```python
from build123d import *

# Parameters (mm, degrees)
F0_W          = 87.5
F0_H          = 92
F1_DEPTH      = 42
F1_TAPER      = 4
F1_DEPTH_BACK = 33
F5_SIZE       = 5
F6_T1_DEPTH   = 58.7168298797
F6_T3_DEPTH   = 62.7898982715
F6_T5_DEPTH   = 62.7898982715
F6_T7_DEPTH   = 62.7898982715
F6_T9_DEPTH   = 62.7898982715
F7_T1_DEPTH   = 103.6905771188
F7_T3_DEPTH   = 44.0479092504
F7_T5_DEPTH   = 44.0479092504
F7_T7_DEPTH   = 108.1905771188
F7_T9_DEPTH   = 44.0479092503
F7_T11_DEPTH  = 44.0479092503


# Not quite as in the source:
# - a fillet or chamfer that OpenCascade refuses, or shapes differently, is made with other operations: its cross-section is extruded or revolved along the edge and cut away or added


with BuildPart() as f1:
    # F0 (on Top) → F1 (new body, two sides)
    with BuildSketch(Plane.XY) as f1_sk:
        with Locations((0, -1.4119595289)):
            Rectangle(F0_W, F0_H)
    extrude(amount=F1_DEPTH, taper=F1_TAPER)
    extrude(f1_sk.sketch, amount=-F1_DEPTH_BACK)

    # F5
    f5_edges = [f1.edges().sort_by_distance(p)[0] for p in [
        (0, -44.475033, 42),
        (40.813074, -1.41196, 42),
        (0, 41.651114, 42),
        (-40.813074, -1.41196, 42),
    ]]
    chamfer(f5_edges, length=F5_SIZE)

    # F6: chamfer of 5 on 8 edges, made by hand

    # F6_s2 → F6_t1 (cut)
    with BuildSketch(Plane.XY.offset(-45.8584149398)):
        Polygon((43.75, 39.5880404711), (38.75, 44.5880404711), (43.75, 44.5880404711), align=None)
        Polygon((-43.75, 39.5880404711), (-38.75, 44.5880404711), (-43.75, 44.5880404711), align=None)
        Polygon((-38.75, -47.4119595289), (-43.75, -42.4119595289), (-43.75, -47.4119595289), align=None)
        Polygon((38.75, -47.4119595289), (43.75, -42.4119595289), (43.75, -47.4119595289), align=None)
    extrude(amount=F6_T1_DEPTH, mode=Mode.SUBTRACT)

    # F6_s4 → F6_t3 (cut)
    with BuildSketch(Plane(origin=(-1.3320626645, -1.3320626645, -19.0493835976), x_dir=(-0.7071067812, 0.7071067812, 0), z_dir=(0.0695873743, 0.0695873743, 0.9951458158))):
        Polygon((-6.1163179384, 60.6385318402), (0.9375251077, 60.6385318402), (-2.5893964153, 64.1483330365), align=None)
    extrude(amount=F6_T3_DEPTH, mode=Mode.SUBTRACT)

    # F6_s6 → F6_t5 (cut)
    with BuildSketch(Plane(origin=(1.3320626645, -1.3320626645, -19.0493835976), x_dir=(-0.7071067812, -0.7071067812, 0), z_dir=(-0.0695873743, 0.0695873743, 0.9951458158))):
        Polygon((6.1163179384, 60.6385318402), (-0.9375251077, 60.6385318402), (2.5893964153, 64.1483330365), align=None)
    extrude(amount=F6_T5_DEPTH, mode=Mode.SUBTRACT)

    # F6_s8 → F6_t7 (cut)
    with BuildSketch(Plane(origin=(-1.3183881113, 1.3183881113, -18.8538283766), x_dir=(0.7071067812, 0.7071067812, 0), z_dir=(0.0695873743, -0.0695873743, 0.9951458158))):
        Polygon((-2.934337423, 58.6514124197), (4.119505623, 58.6514124197), (0.5925841, 62.161213616), align=None)
    extrude(amount=F6_T7_DEPTH, mode=Mode.SUBTRACT)

    # F6_s10 → F6_t9 (cut)
    with BuildSketch(Plane(origin=(1.3183881113, 1.3183881113, -18.8538283766), x_dir=(0.7071067812, -0.7071067812, 0), z_dir=(-0.0695873743, -0.0695873743, 0.9951458158))):
        Polygon((2.934337423, 58.6514124197), (-4.119505623, 58.6514124197), (-0.5925841, 62.161213616), align=None)
    extrude(amount=F6_T9_DEPTH, mode=Mode.SUBTRACT)

    # F7: fillet of radius 150 on 8 edges, made by hand

    # F7_s2 → F7_t1 (cut)
    with BuildSketch(Plane.YZ.offset(-51.8452885594)):
        with BuildLine():
            ThreePointArc((-47.0465670679, 5.2253556379), (-47.3205835818, -0.0031909184), (-47.4119595289, -5.2381154238))
            Line((-47.4119595289, -5.2381154238), (-47.4119595289, 0))
            Line((-47.4119595289, 0), (-47.0465670679, 5.2253556379))
        make_face()
        with BuildLine():
            ThreePointArc((44.5880404711, -5.2381154238), (44.4966645239, -0.0031909184), (44.2226480101, 5.2253556379))
            Line((44.2226480101, 5.2253556379), (44.5880404711, 0))
            Line((44.5880404711, 0), (44.5880404711, -5.2381154238))
        make_face()
    extrude(amount=F7_T1_DEPTH, mode=Mode.SUBTRACT)

    # F7_s4 → F7_t3 (cut)
    with BuildSketch(Plane(origin=(13.7423078996, 13.7423078996, 0), x_dir=(0, 0, 1), z_dir=(-0.7071067812, -0.7071067812, 0))):
        with BuildLine():
            ThreePointArc((-7.3117239806, -60.9257058632), (0.078105005, -60.7435633688), (7.4499872987, -60.1975782307))
            Line((7.4499872987, -60.1975782307), (0.0870892603, -60.9257058632))
            Line((0.0870892603, -60.9257058632), (-7.3117239806, -60.9257058632))
        make_face()
    extrude(amount=F7_T3_DEPTH, mode=Mode.SUBTRACT)

    # F7_s6 → F7_t5 (cut)
    with BuildSketch(Plane(origin=(17.4042674285, -17.4042674285, 0), x_dir=(0, 0, 1), z_dir=(-0.7071067812, 0.7071067812, 0))):
        with BuildLine():
            ThreePointArc((7.4499872987, -60.1975782307), (0.078105005, -60.7435633688), (-7.3117239806, -60.9257058632))
            Line((-7.3117239806, -60.9257058632), (0.0870892603, -60.9257058632))
            Line((0.0870892603, -60.9257058632), (7.4499872987, -60.1975782307))
        make_face()
    extrude(amount=F7_T5_DEPTH, mode=Mode.SUBTRACT)

    # F7_s8 → F7_t7 (cut)
    with BuildSketch(Plane.XZ.offset(-52.6833290305)):
        with BuildLine():
            ThreePointArc((43.75, -5.2381154238), (43.6586240529, -0.0031909184), (43.384607539, 5.2253556379))
            Line((43.384607539, 5.2253556379), (43.75, 0))
            Line((43.75, 0), (43.75, -5.2381154238))
        make_face()
        with BuildLine():
            ThreePointArc((-43.384607539, 5.2253556379), (-43.6586240529, -0.0031909184), (-43.75, -5.2381154238))
            Line((-43.75, -5.2381154238), (-43.75, 0))
            Line((-43.75, 0), (-43.384607539, 5.2253556379))
        make_face()
    extrude(amount=F7_T7_DEPTH, mode=Mode.SUBTRACT)

    # F7_s10 → F7_t9 (cut)
    with BuildSketch(Plane(origin=(-15.1542674285, -15.1542674285, 0), x_dir=(0, 0, 1), z_dir=(0.7071067812, 0.7071067812, 0))):
        with BuildLine():
            ThreePointArc((-7.3117239809, -58.9288935479), (0.0781050046, -58.7467510535), (7.4499872984, -58.2007659154))
            Line((7.4499872984, -58.2007659154), (0.08708926, -58.9288935479))
            Line((0.08708926, -58.9288935479), (-7.3117239809, -58.9288935479))
        make_face()
    extrude(amount=F7_T9_DEPTH, mode=Mode.SUBTRACT)

    # F7_s12 → F7_t11 (cut)
    with BuildSketch(Plane(origin=(-15.9923078995, 15.9923078995, 0), x_dir=(0, 0, 1), z_dir=(0.7071067812, -0.7071067812, 0))):
        with BuildLine():
            ThreePointArc((-7.3117239809, -58.9288935479), (0.0781050046, -58.7467510535), (7.4499872984, -58.2007659154))
            Line((7.4499872984, -58.2007659154), (0.08708926, -58.9288935479))
            Line((0.08708926, -58.9288935479), (-7.3117239809, -58.9288935479))
        make_face()
    extrude(amount=F7_T11_DEPTH, mode=Mode.SUBTRACT)


solid = f1.part
```
Can you work these out from the model? Positions are in its coordinate system, mm. Coordinates: 2 decimals unless noted, no trailing zeros. Loops run counter-clockwise (first coordinate to the right, second up) from the corner with the lowest first, then second, coordinate; pieces in that order, holes last.
1) Imagine slicing it at C-C on z = 13.5. List the corners of the cut face in (x, y) for me.
2) Imagine slicing it at B-B on y = -2. List the corners of the cut face in (x, z) for me, plus the area to 3 significant figures.
3) Imagine slicing it at A-A on x = 10. List the corners of the cut face in (y, z) for me.
4) For pin 1 (3 mm diameter, centred on y = -16, z = -4.5, fed in from -X); pin 2 (10 mm diameter, centred on y = -6, z = 20.5, fed in from +X); pin 3 (5 mm diameter, centred on y = -8, z = 28.5, fed in from -X); pin 4 (8 mm diameter, centred on y = 14, z = 20.5, fed in from -X), each with a flat end and sliding along its axis, tell me the tip position at first contact or that it passes through.
5) I need wall thicknesses on probe 1 along X at (y, z) = (3, 32); probe 2 along Y at (x, z) = (-13, 28); probe 3 along X at (y, z) = (-42, 14). Which ranges of each line are inside material? Lowest first, please.
Completed:
1. outline: (-42.81, -41.48) - (-37.82, -46.47) - (37.82, -46.47) - (42.81, -41.48) - (42.81, 38.66) - (37.82, 43.64) - (-37.82, 43.64) - (-42.81, 38.66) - close
2. outline: (-43.75, -33) - (43.75, -33) - (43.75, -5.24) arc R150 ccw to (43.38, 5.23) - (41.16, 37.01) - (35.81, 42) - (-35.81, 42) - (-41.16, 37.01) - (-43.38, 5.23) arc R150 ccw to (-43.75, -5.24) - close
2. area: 6,410 mm2
3. outline: (-47.41, -33) - (44.59, -33) - (44.59, -5.24) arc R150 ccw to (44.22, 5.23) - (42, 37.01) - (36.65, 42) - (-39.48, 42) - (-44.82, 37.01) - (-47.05, 5.23) arc R150 ccw to (-47.41, -5.24) - close
4. pin 1: stops at x = -43.75
4. pin 2: stops at x = 42.67
4. pin 3: stops at x = -41.93
4. pin 4: stops at x = -42.6
5. probe 1: x = -41.51 to 41.51
5. probe 2: y = -45.45 to 42.63
5. probe 3: x = -42.22 to 42.22
